The model under review builds one solid part; all positions refer to its coordinate system, in mm. Face numbers are marked on the shaded views. A direction names the side the tool comes from. Coordinates: 2 decimals unless noted, no trailing zeros. Write each loop counter-clockwise with the first axis right and the second up, starting at its lowest first coordinate (ties: lowest second). Pieces come first, ordered by that corner, then holes.
```python
from build123d import *

# Parameters (mm, degrees)
SKETCH1_W           = 4.826
SKETCH1_H           = 3.96875
SKETCH2_R           = 2.413
BOSS_EXTRUDE1_DEPTH = 12.7
CUT_EXTRUDE1_DEPTH  = 2.286
CHAMFER1_SIZE       = 0.47244
FILLET1_R           = 0.3556


with BuildPart() as part:
    # Sketch1 → Revolve1 (revolve)
    with BuildSketch(Plane(origin=(0, 0, 0), x_dir=(-1, 0, 0), z_dir=(0, 0, -1)), mode=Mode.PRIVATE) as revolve1_sk:
        with Locations((-2.413, 1.984375)):
            Rectangle(SKETCH1_W, SKETCH1_H)
    revolve(revolve1_sk.sketch.rotate(Axis((4.826, 0, 0), (-1, 0, 0)), 270), axis=Axis((4.826, 0, 0), (-1, 0, 0)))

    # Sketch2 → Boss-Extrude1 (add)
    with BuildSketch(Plane(origin=(4.826, 0, 0), x_dir=(0, 0, -1), z_dir=(1, 0, 0))):
        Circle(SKETCH2_R)
    extrude(amount=BOSS_EXTRUDE1_DEPTH)

    # Sketch3 → Cut-Extrude1 (cut)
    with BuildSketch(Plane.ZY):
        Polygon((0, -2.292092116), (1.98501, -1.146046058), (1.98501, 1.146046058), (0, 2.292092116), (-1.98501, 1.146046058), (-1.98501, -1.146046058), align=None)
    extrude(amount=-CUT_EXTRUDE1_DEPTH, mode=Mode.SUBTRACT)

    # Sketch4 → Cut-Revolve1 (revolve, cut)
    with BuildSketch(Plane.XY, mode=Mode.PRIVATE) as cut_revolve1_sk:
        Polygon((2.286, 1.98501), (2.286, 0), (3.432046058, 0), align=None)
    revolve(cut_revolve1_sk.sketch.rotate(Axis((2.286, 0, 0), (1, 0, 0)), 90), axis=Axis((2.286, 0, 0), (1, 0, 0)), mode=Mode.SUBTRACT)

    # Chamfer1
    chamfer1_edges = [part.edges().sort_by_distance(p)[0] for p in [
        (0, 0, -3.96875),
        (17.526, 0, 2.413),
    ]]
    chamfer(chamfer1_edges, length=CHAMFER1_SIZE)

    # Fillet1
    fillet1_edges = [part.edges().sort_by_distance(p)[0] for p in [
        (4.826, 0, 2.413),
    ]]
    fillet(fillet1_edges, radius=FILLET1_R)


solid = part.part
```
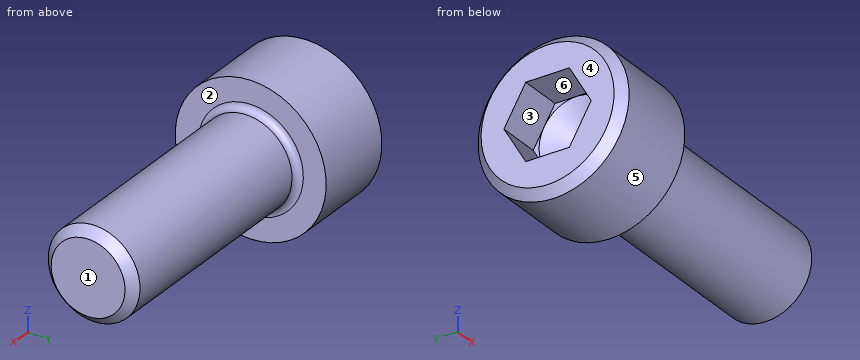
Item 1: For pin 1 (0.5 mm diameter, centred on y = -1, z = -1.5, fed in from -X); pin 2 (0.7 mm diameter, centred on x = 1.5, y = 0.5, fed in from +Z); pin 3 (2 mm diameter, centred on x = 5, z = 3, fed in from +Y), all flat-tipped, find the tip position at first contact; note any pin that passes through.
Solved:
pin 1: stops at x = 2.29
pin 2: stops at z = 3.97
pin 3: stops at y = 3.42
Item 2: Mouldability with a two-part tool opening along Z and no side actions: class the marked faces 4, 5 and 6 as pulls with the +Z half, pulls with the -Z half, needs draft (parallel to the pull), parting line crosses it, or undercut.
Solved:
face 4: needs draft
face 5: parting line crosses it
face 6: undercut
Item 3: Take a section at A-A, the plane x = 1. Write out the cut boundary in (y, z), plus the area to 3 significant figures.
Solved:
outline: circle Ø7.94 at (0, 0); hole (-2.29, 0) - (-1.15, -1.99) - (1.15, -1.99) - (2.29, 0) - (1.15, 1.99) - (-1.15, 1.99) - close
area: 35.8 mm2
Item 4: Take a section at B-B, the plane x = 7.5. Write out the cut boundary in (y, z), plus the area to 3 significant figures.
Solved:
outline: circle Ø4.83 at (0, 0)
area: 18.3 mm2
Item 5: Machinability: for the marked faces 1, 2 and 3, which of the approach directions +Z, -Z, +X, -X, +Y, -Y give a long, thin tool a straight path to every point of the face, cutting with its end or side? Answer none if there is none.
Solved:
face 1: +Z, -Z, +X, +Y, -Y
face 2: +X
face 3: -X
Item 6: To check wall thickness, follow line 1 along Y through (x, z) = (1, 1); line 2 along Y through (x, z) = (3, 0.5); line 3 along Z through (x, y) = (2.75, -0.5). State the ranges of each line that lie inside material, in increasing order.
Solved:
line 1: y = -3.84 to -1.71, 1.71 to 3.84
line 2: y = -3.94 to -0.56, 0.56 to 3.94
line 3: z = -3.94 to -1.07, 1.07 to 3.94
